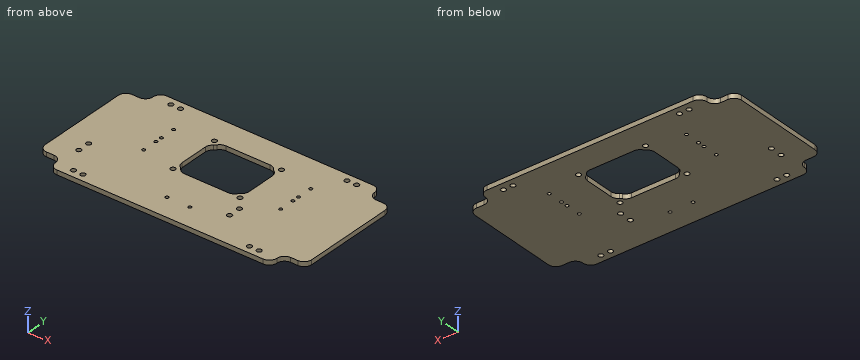
Autodesk Inventor part; units mm, degrees
ref_plane "YZ Plane" through (0, 0, 0) normal (1, 0, 0) x (0, 1, 0)
ref_plane "XZ Plane" through (0, 0, 0) normal (0, 1, 0) x (-1, 0, 0)
ref_plane "XY Plane" through (0, 0, 0) normal (0, 0, 1) x (1, 0, 0)
sketch "スケッチ1" plane through (0, 0, 0) normal (0, 0, 1) x (1, 0, 0)
  line L0 (-96.735, 64.25) -> (78.265, 64.25)
  line L1 (78.265, 64.25) -> (78.265, -25.75)
  line L2 (78.265, -25.75) -> (-96.735, -25.75)
  line L3 (-96.735, -25.75) -> (-96.735, 64.25)
  line L4 (-96.735, 64.25) -> (78.265, -25.75) construction
  line L5 (78.265, 64.25) -> (-96.735, -25.75) construction
  line L6 (-96.735, 19.25) -> (78.265, 19.25) construction
  line L7 (-96.735, 0) -> (78.265, 0) construction
  line L8 (-80, 4) -> (-80, -4) construction
  circle A0 centre (-80, -4) radius 1.6
  line L9 (0, 64.25) -> (0, -25.75) construction
  line L10 (19, -4) -> (19, 4) construction
  circle A1 centre (19, -4) radius 1.6
  circle A2 centre (-80, 4) radius 1.6
  circle A3 centre (19, 4) radius 1.6
  line L11 (16, 12.5) -> (22, 12.5) construction
  line L12 (22, 12.5) -> (22, -12.5) construction
  line L13 (22, -12.5) -> (16, -12.5) construction
  line L14 (16, -12.5) -> (16, 12.5) construction
  line L15 (16, 12.5) -> (22, -12.5) construction
  line L16 (22, 12.5) -> (16, -12.5) construction
  line L17 (-83, 12.5) -> (-77, 12.5) construction
  line L18 (-77, 12.5) -> (-77, -12.5) construction
  line L19 (-77, -12.5) -> (-83, -12.5) construction
  line L20 (-83, -12.5) -> (-83, 12.5) construction
  line L21 (-83, 12.5) -> (-77, -12.5) construction
  line L22 (-77, 12.5) -> (-83, -12.5) construction
  line L23 (-67, 49.25) -> (6, 49.25) construction
  line L24 (6, 49.25) -> (6, -10.75) construction
  line L25 (6, -10.75) -> (-67, -10.75) construction
  line L26 (-67, -10.75) -> (-67, 49.25) construction
  line L27 (-67, 49.25) -> (6, -10.75) construction
  line L28 (6, 49.25) -> (-67, -10.75) construction
  line L29 (-83, -4.5) -> (-83, 20.5) construction
  line L30 (-83, 20.5) -> (-77, 20.5) construction
  line L31 (-77, 20.5) -> (-77, -4.5) construction
  line L32 (-77, -4.5) -> (-83, -4.5) construction
  circle A4 centre (-80, 12) radius 1.6
  circle A5 centre (-80, 4) radius 1.6
  line L33 (16, 20.5) -> (22, 20.5) construction
  line L34 (16, -4.5) -> (16, 20.5) construction
  line L35 (22, -4.5) -> (16, -4.5) construction
  line L36 (22, 20.5) -> (22, -4.5) construction
  circle A6 centre (19, 4) radius 1.6
  circle A7 centre (19, 12) radius 1.6
  line L37 (-83, 3.5) -> (-83, 28.5) construction
  line L38 (-83, 28.5) -> (-77, 28.5) construction
  line L39 (-77, 28.5) -> (-77, 3.5) construction
  line L40 (-77, 3.5) -> (-83, 3.5) construction
  circle A8 centre (-80, 20) radius 1.6
  circle A9 centre (-80, 12) radius 1.6
  line L41 (16, 28.5) -> (22, 28.5) construction
  line L42 (16, 3.5) -> (16, 28.5) construction
  line L43 (22, 3.5) -> (16, 3.5) construction
  line L44 (22, 28.5) -> (22, 3.5) construction
  circle A10 centre (19, 12) radius 1.6
  circle A11 centre (19, 20) radius 1.6
  circle A12 centre (-80, -12) radius 1.6
  line L45 (-77, -20.5) -> (-83, -20.5) construction
  line L46 (-83, -20.5) -> (-83, 4.5) construction
  line L47 (-77, 4.5) -> (-77, -20.5) construction
  line L48 (16, -20.5) -> (16, 4.5) construction
  circle A13 centre (19, -12) radius 1.6
  line L49 (22, -20.5) -> (16, -20.5) construction
  line L50 (22, 4.5) -> (22, -20.5) construction
  line L51 (45.415, -24.7) -> (77.215, -24.7) construction
  line L52 (77.215, -16.8) -> (45.415, -16.8) construction
  line L53 (45.415, -16.8) -> (45.415, -24.7) construction
  line L54 (45.415, -24.7) -> (77.215, -16.8) construction
  line L55 (77.215, -24.7) -> (45.415, -16.8) construction
  line L56 (77.215, -20.75) -> (45.415, -20.75) construction
  line L57 (61.315, -24.7) -> (61.315, -16.8) construction
  circle A14 centre (45.415, -20.75) radius 1.6
  circle A15 centre (51.765, -20.75) radius 1.6
  line L58 (73.615, -19.1623) -> (73.615, -22.3377) construction
  line L59 (73.615, -22.3377) -> (70.865, -23.9254) construction
  line L60 (70.865, -23.9254) -> (68.115, -22.3377) construction
  line L61 (68.115, -22.3377) -> (68.115, -19.1623) construction
  line L62 (68.115, -19.1623) -> (70.865, -17.5746) construction
  line L63 (70.865, -17.5746) -> (73.615, -19.1623) construction
  line L64 (-9.235, 64.25) -> (-9.235, -25.75) construction
  circle A16 centre (45.415, 59.25) radius 1.6
  circle A17 centre (51.765, 59.25) radius 1.6
  line L65 (73.615, 57.6623) -> (73.615, 60.8377) construction
  line L66 (73.615, 60.8377) -> (70.865, 62.4254) construction
  line L67 (70.865, 62.4254) -> (68.115, 60.8377) construction
  line L68 (68.115, 60.8377) -> (68.115, 57.6623) construction
  line L69 (68.115, 57.6623) -> (70.865, 56.0746) construction
  line L70 (70.865, 56.0746) -> (73.615, 57.6623) construction
  circle A18 centre (-63.885, -20.75) radius 1.6
  circle A19 centre (-70.235, -20.75) radius 1.6
  line L71 (-92.085, -19.1623) -> (-92.085, -22.3377) construction
  line L72 (-92.085, -22.3377) -> (-89.335, -23.9254) construction
  line L73 (-89.335, -23.9254) -> (-86.585, -22.3377) construction
  line L74 (-86.585, -22.3377) -> (-86.585, -19.1623) construction
  line L75 (-86.585, -19.1623) -> (-89.335, -17.5746) construction
  line L76 (-89.335, -17.5746) -> (-92.085, -19.1623) construction
  circle A20 centre (-63.885, 59.25) radius 1.6
  circle A21 centre (-70.235, 59.25) radius 1.6
  line L77 (-86.585, 57.6623) -> (-89.335, 56.0746) construction
  line L78 (-86.585, 60.8377) -> (-86.585, 57.6623) construction
  line L79 (-89.335, 62.4254) -> (-86.585, 60.8377) construction
  line L80 (-92.085, 60.8377) -> (-89.335, 62.4254) construction
  line L81 (-92.085, 57.6623) -> (-92.085, 60.8377) construction
  line L82 (-89.335, 56.0746) -> (-92.085, 57.6623) construction
  line L83 (-34.235, 49.25) -> (15.765, 49.25) construction
  line L84 (15.765, 49.25) -> (15.765, 9.25) construction
  line L85 (15.765, 9.25) -> (-34.235, 9.25) construction
  line L86 (-34.235, 9.25) -> (-34.235, 49.25) construction
  line L87 (-34.235, 49.25) -> (15.765, 9.25) construction
  line L88 (15.765, 49.25) -> (-34.235, 9.25) construction
  line L89 (-31.235, 46.25) -> (12.765, 46.25) construction
  line L90 (12.765, 46.25) -> (12.765, 12.25) construction
  line L91 (12.765, 12.25) -> (-31.235, 12.25) construction
  line L92 (-31.235, 12.25) -> (-31.235, 46.25) construction
  line L93 (-31.235, 46.25) -> (12.765, 12.25) construction
  line L94 (12.765, 46.25) -> (-31.235, 12.25) construction
  circle A22 centre (-31.235, 12.25) radius 1.6
  circle A23 centre (-31.235, 46.25) radius 1.6
  circle A24 centre (12.765, 46.25) radius 1.6
  circle A25 centre (12.765, 12.25) radius 1.6
  line L95 (-62, -21.85) -> (-61.735, -21.85)
  line L96 (77.215, -16.8) -> (77.215, -24.7) construction
  line L97 (63.465, -25.75) -> (63.465, -15.75)
  line L98 (63.465, -15.75) -> (78.265, -15.75)
  line L99 (70.865, -23.9254) -> (70.865, -17.5746) construction
  line L100 (63.465, 64.25) -> (63.465, 54.25)
  line L101 (63.465, 54.25) -> (78.265, 54.25)
  line L102 (-81.935, -25.75) -> (-81.935, -15.75)
  line L103 (-81.935, -15.75) -> (-96.735, -15.75)
  line L104 (-81.935, 54.25) -> (-96.735, 54.25)
  line L105 (-81.935, 64.25) -> (-81.935, 54.25)
  line L106 (-9.235, 49.25) -> (-9.235, 9.25) construction
  circle A26 centre (35.765, 31.5525) radius 1.05
  circle A27 centre (35.765, 41.5525) radius 1.05
  line L107 (35.765, 31.5525) -> (35.765, 41.5525) construction
  line L108 (-34.235, 29.25) -> (15.765, 29.25) construction
  circle A28 centre (35.765, 26.9475) radius 1.05
  circle A29 centre (35.765, 16.9475) radius 1.05
  circle A30 centre (-54.235, 31.5525) radius 1.05
  circle A31 centre (-54.235, 41.5525) radius 1.05
  circle A32 centre (-54.235, 26.9475) radius 1.05
  circle A33 centre (-54.235, 16.9475) radius 1.05
  circle A34 centre (-16.735, -10.75) radius 1.05
  circle A35 centre (-1.735, -10.75) radius 1.05
  line L109 (-1.735, -10.75) -> (-16.735, -10.75) construction
  arc A36 (-27.235, 12.25) -> (-31.235, 16.25) centre (-31.235, 12.25) ccw
  line L110 (-31.235, 16.25) -> (-31.235, 42.25)
  line L111 (-27.235, 12.25) -> (8.765, 12.25)
  arc A37 (12.765, 16.25) -> (8.765, 12.25) centre (12.765, 12.25) ccw
  line L112 (12.765, 16.25) -> (12.765, 42.25)
  arc A38 (-31.235, 42.25) -> (-27.235, 46.25) centre (-31.235, 46.25) ccw
  line L113 (-27.235, 46.25) -> (8.765, 46.25)
  arc A39 (8.765, 46.25) -> (12.765, 42.25) centre (12.765, 46.25) ccw
  point P0 (0, 0)
  point P1 (-9.235, 19.25)
  point P2 (-80, 0)
  point P3 (19, 0)
  point P4 (-30.5, 19.25)
  point P5 (61.315, -20.75)
  point P6 (70.865, -20.75)
  point P7 (-9.235, 29.25)
  point P8 (-9.235, 29.25)
  point P9 (-9.235, 29.25)
  point P10 (35.765, 36.5525)
  point P11 (-9.235, -10.75)
  dimension "d0" = 175
  dimension "d1" = 90
  dimension "d2" = 25.75
  dimension "d3" = 3.2
  dimension "d4" = 8
  dimension "d5" = 8
  dimension "d6" = 3.2
  dimension "d16" = 78.265
  dimension "d17" = 6
  dimension "d18" = 25
  dimension "d19" = 22
  dimension "d20" = 6
  dimension "d21" = 25
  dimension "d22" = 105
  dimension "d23" = 15
  dimension "d24" = 15
  dimension "d25" = 10
  dimension "d26" = 10
  dimension "d57" = 8
  dimension "d64" = 8
  dimension "d69" = 31.8
  dimension "d70" = 7.9
  dimension "d72" = 3.2
  dimension "d75" = 5.5
  dimension "d79" = 50
  dimension "d80" = 40
  dimension "d81" = 44
  dimension "d82" = 34
  dimension "d83" = 3.2
  dimension "d88" = 10
  dimension "d89" = 87.5
  dimension "d102" = 19.1
  dimension "d103" = 5
  dimension "d104" = 1.05
  dimension "d105" = 7.4
  dimension "d106" = 1.05
  dimension "d107" = 2.1
  dimension "d109" = 20
  dimension "d110" = 10
  dimension "d111" = 7.3025
  dimension "d112" = 42.765
  dimension "d113" = 10
  dimension "d114" = 15
  dimension "d115" = 20
  dimension "d116" = 4
extrude "押し出し1" add sketch "スケッチ1" along normal blind 3 contours L0 L100 L101 L1 L98 L97 L2 L102 L103 L3 L104 L105 | A4 | A7 | A8 | A11 | A12 | A13
fillet "フィレット1" radius 5 20 edges at (-81.935, -25.75, 1.5) (-81.935, -15.75, 1.5) (-96.735, -15.75, 1.5) (-96.735, 54.25, 1.5) (-81.935, 54.25, 1.5) (-81.935, 64.25, 1.5) (63.465, 64.25, 1.5) (63.465, 54.25, 1.5) (78.265, 54.25, 1.5) (78.265, -15.75, 1.5) (63.465, -25.75, 1.5) (63.465, -15.75, 1.5) (-27.235, 12.25, 1.5) (-31.235, 16.25, 1.5) (-31.235, 42.25, 1.5) (-27.235, 46.25, 1.5) (8.765, 46.25, 1.5) (12.765, 42.25, 1.5) (12.765, 16.25, 1.5) (8.765, 12.25, 1.5)
equation "\"d3\" = d6"
equation "\"d4\" = d5"
equation "\"d20\" = d17"
equation "\"d21\" = d18"
properties part number "Sole_frame" material "GFRP"
The listing builds one solid part. Answer for the finished solid, in the listing's coordinates (mm). Round coordinates to 2 decimals unless told otherwise and drop trailing zeros. Write each loop counter-clockwise with the first axis right and the second up, starting at its lowest first coordinate (ties: lowest second). Pieces come first, ordered by that corner, then holes. Notation, with made-up numbers: M 50.5,57 L 80.5,57 A36 cw 80.5,91 Z; hole C 18.5,-13.5 d5. An arc over 180 degrees is marked long. Write each question's results on one line, items separated by ' | '. Start each with the question number.
(1) Each of these flat-tipped pins is pushed along its axis until it touches: P1, Ø1.7, axis at x = 35.76, y = 41.55, coming from the -Z side; P2, Ø1.5, axis at x = 70.5, z = 2, coming from the +Y side; P3, Ø1, axis at y = -14, z = 1, coming from the -X side; P4, Ø1.5, axis at x = -88, z = 1.5, coming from the -Y side. Where does it stop, or does it pass through?
(2) The part is cut by section C-C, the plane y = -4. Write down the section's boundary in (x, z) (3 decimals).
(3) Find the intervals of material crossed by line 1 (X direction, y = -20.5, z = 0.65); line 2 (X direction, y = 36, z = 2) (3 decimals); line 3 (Y direction, x = -22, z = 2.25), in increasing order.
(4) The part is cut by section A-A, the plane y = 36.5. Write down the section's boundary in (x, z) (3 decimals).
(5) The part is cut by section B-B, the plane x = 19. Write down the section's boundary in (y, z).
(6) The part is cut by section D-D, the plane z = 0.5. Give the number of separate pieces and of enclosed holes in the cut face, and give its area (3 significant figures).
Worked answers:
1) P1: passes through | P2: stops at y = 54.25 | P3: stops at x = -95.91 | P4: stops at y = -15.75
2) outline: M -96.735,0 L -81.6,0 L -81.6,3 L -96.735,3 Z; M -78.4,0 L 17.4,0 L 17.4,3 L -78.4,3 Z; M 20.6,0 L 78.265,0 L 78.265,3 L 20.6,3 Z
3) line 1: x = -81.94 to -71.82, -68.65 to -65.47, -62.3 to 43.83, 47 to 50.18, 53.35 to 63.47 | line 2: x = -96.735 to -31.235, 12.765 to 78.265 | line 3: y = -25.75 to 12.25, 46.25 to 64.25
4) outline: M -96.735,0 L -31.235,0 L -31.235,3 L -96.735,3 Z; M 12.765,0 L 78.265,0 L 78.265,3 L 12.765,3 Z
5) outline: M -25.75,0 L -5.6,0 L -5.6,3 L -25.75,3 Z; M -2.4,0 L 2.4,0 L 2.4,3 L -2.4,3 Z; M 5.6,0 L 64.25,0 L 64.25,3 L 5.6,3 Z
6) separate pieces: 1 | enclosed holes: 27 | area: 13,500 mm²
